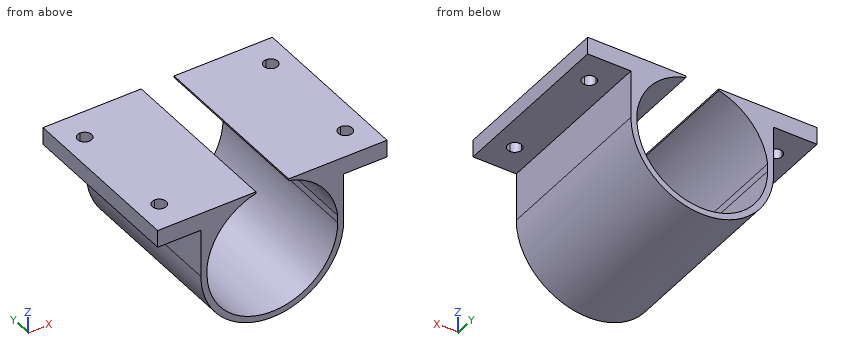
```python
from build123d import *

# Parameters (mm, degrees)
BOSS_EXTRUDE3_DEPTH = 40
SKETCH8_W           = 4
SKETCH8_H           = 40
BOSS_EXTRUDE6_DEPTH = 10
SKETCH9_W           = 4
SKETCH9_H           = 40
BOSS_EXTRUDE7_DEPTH = 10
BOSS_EXTRUDE9_DEPTH = 40
CUT_EXTRUDE1_DEPTH  = 40
SCALE1_SCALE_X      = 0.8
SCALE1_SCALE_Y      = 0.8
SCALE1_SCALE_Z      = 0.8


with BuildPart() as part:
    # Sketch3 → Boss-Extrude3 (new body)
    with BuildSketch(Plane(origin=(0, 0, 0), x_dir=(1, 0, 0), z_dir=(0, 1, 0))):
        with BuildLine():
            ThreePointArc((16.5, 0), (0, 16.5), (-16.5, 0))
            Line((-16.5, 0), (-16.5, -15.1))
            Line((-16.5, -15.1), (-15.1, -15.1))
            Line((-15.1, -15.1), (-15.1, 0))
            ThreePointArc((-15.1, 0), (0, 15.1), (15.1, 0))
            Line((15.1, 0), (15.1, -15.1))
            Line((15.1, -15.1), (16.5, -15.1))
            Line((16.5, -15.1), (16.5, 0))
        make_face()
    extrude(amount=BOSS_EXTRUDE3_DEPTH)

    # Sketch8 → Boss-Extrude6 (add)
    with BuildSketch(Plane(origin=(16.5, 0, 0), x_dir=(0, 0, -1), z_dir=(1, 0, 0))):
        with Locations((-13.1, 20)):
            Rectangle(SKETCH8_W, SKETCH8_H)
    extrude(amount=BOSS_EXTRUDE6_DEPTH)

    # Sketch9 → Boss-Extrude7 (add)
    with BuildSketch(Plane.ZY.offset(16.5)):
        with Locations((13.1, 20)):
            Rectangle(SKETCH9_W, SKETCH9_H)
    extrude(amount=BOSS_EXTRUDE7_DEPTH)

    # Sketch10 → Boss-Extrude9 (add)
    with BuildSketch(Plane(origin=(0, 0, 0), x_dir=(-1, 0, 0), z_dir=(0, -1, 0))):
        with BuildLine():
            Line((3.791332709, -15.1), (15.1, -15.1))
            Line((15.1, -15.1), (15.1, -1.740689519))
            ThreePointArc((15.1, -1.740689519), (11.460081139, -9.985316234), (3.791332709, -14.719571879))
            Line((3.791332709, -14.719571879), (3.791332709, -15.1))
        make_face()
        with BuildLine():
            Line((-15.1, -15.1), (-3.791332709, -15.1))
            Line((-3.791332709, -15.1), (-3.791332709, -14.719571879))
            ThreePointArc((-3.791332709, -14.719571879), (-11.460081139, -9.985316234), (-15.1, -1.740689519))
            Line((-15.1, -1.740689519), (-15.1, -15.1))
        make_face()
    extrude(amount=-BOSS_EXTRUDE9_DEPTH)

    # Sketch11 → Cut-Extrude1 (cut)
    with BuildSketch(Plane(origin=(0, 0, 11.1), x_dir=(-1, 0, 0), z_dir=(0, 0, -1))):
        with BuildLine():
            ThreePointArc((-19.9, 33), (-20.36862915, 34.13137085), (-21.5, 34.6))
            Line((-21.5, 34.6), (-21.5, 31.4))
            ThreePointArc((-21.5, 31.4), (-20.36862915, 31.86862915), (-19.9, 33))
        make_face()
        with BuildLine():
            Line((-21.5, 31.4), (-21.5, 34.6))
            ThreePointArc((-21.5, 34.6), (-23.1, 33), (-21.5, 31.4))
        make_face()
        with BuildLine():
            ThreePointArc((-19.9, 7), (-20.36862915, 8.13137085), (-21.5, 8.6))
            Line((-21.5, 8.6), (-21.5, 5.4))
            ThreePointArc((-21.5, 5.4), (-20.36862915, 5.86862915), (-19.9, 7))
        make_face()
        with BuildLine():
            Line((-21.5, 5.4), (-21.5, 8.6))
            ThreePointArc((-21.5, 8.6), (-23.1, 7), (-21.5, 5.4))
        make_face()
        with BuildLine():
            ThreePointArc((23.1, 7), (22.63137085, 8.13137085), (21.5, 8.6))
            Line((21.5, 8.6), (21.5, 5.4))
            ThreePointArc((21.5, 5.4), (22.63137085, 5.86862915), (23.1, 7))
        make_face()
        with BuildLine():
            Line((21.5, 5.4), (21.5, 8.6))
            ThreePointArc((21.5, 8.6), (19.9, 7), (21.5, 5.4))
        make_face()
        with BuildLine():
            ThreePointArc((23.1, 33), (22.63137085, 34.13137085), (21.5, 34.6))
            Line((21.5, 34.6), (21.5, 31.4))
            ThreePointArc((21.5, 31.4), (22.63137085, 31.86862915), (23.1, 33))
        make_face()
        with BuildLine():
            Line((21.5, 31.4), (21.5, 34.6))
            ThreePointArc((21.5, 34.6), (19.9, 33), (21.5, 31.4))
        make_face()
    extrude(amount=-CUT_EXTRUDE1_DEPTH, mode=Mode.SUBTRACT)


with BuildPart() as part_1:
    # Scale1: scaled about (0, 0, 0)
    add(part.part.scale((SCALE1_SCALE_X, SCALE1_SCALE_Y, SCALE1_SCALE_Z), about=(0, 0, 0)))


solid = part_1.part
```
Verification items for the finished model (mm, model axes). Give positions to 0.01 mm unless a question says otherwise; leave off trailing zeros. One line per item, written item: value.
(1) Sectioned sample at A-A on x = -18. Count the separate pieces of the cut face and the enclosed holes in it, then the cut area to 3 significant figures.
Final values:
separate pieces: 3
enclosed holes: 0
area: 89.6 mm^2
(2) Gauge pin test, flat ends, axial feed: pin 1 (12 mm diameter, centred on y = 18.5, z = -2.5, fed in from +X); pin 2 (1.5 mm diameter, centred on y = 27, z = 8, fed in from -X); pin 3 (3 mm diameter, centred on y = 8.5, z = -4.5, fed in from +X). Record the tip position at first contact, or that the pin passes through.
Final values:
pin 1: x = 13.2
pin 2: x = -13.2
pin 3: x = 12.85
(3) Scan lines: line 1 along Z through (x, y) = (16, 23); line 2 along Z through (x, y) = (4, 30); line 3 along X through (y, z) = (6, 7.5). Record each from-to range of solid material in increasing order. Write a range as [from, to].
Final values:
line 1: [8.88, 12.08]
line 2: [-12.58, -11.4], [11.48, 12.08]
line 3: [-13.2, -9.57], [9.57, 13.2]
